Autodesk Inventor part; units mm, degrees
ref_plane "YZ Plane" through (0, 0, 0) normal (1, 0, 0) x (0, 1, 0)
ref_plane "XZ Plane" through (0, 0, 0) normal (0, 1, 0) x (-1, 0, 0)
ref_plane "XY Plane" through (0, 0, 0) normal (0, 0, 1) x (1, 0, 0)
sketch "Sketch1" plane through (0, 0, 0) normal (0, 1, 0) x (-1, 0, 0)
  line L0 (12.7, 25.4) -> (-12.7, 25.4)
  line L1 (-12.7, 25.4) -> (-12.7, -25.4)
  line L2 (-12.7, -25.4) -> (12.7, -25.4)
  line L3 (12.7, -25.4) -> (12.7, 25.4)
  line L4 (12.7, 25.4) -> (-12.7, -25.4) construction
  line L5 (-12.7, 25.4) -> (12.7, -25.4) construction
  point P0 (0, 0)
  dimension "d0" = 25.4
  dimension "d1" = 50.8
extrude "Extrusion1" add sketch "Sketch1" along normal blind 6.35
sketch "Sketch3" plane through (12.7, 0, 25.4) normal (1, 0, 0) x (0, 0, -1)
  line L0 (0, 6.35) -> (50.8, 6.35)
  line L1 (50.8, 6.35) -> (25.4, 6.35)
  line L2 (25.4, 6.35) -> (25.4, 0)
  line L3 (25.4, 0) -> (50.8, 0)
  line L4 (50.8, 0) -> (50.8, 6.35)
  dimension "d14" = 25.4
extrude "Extrusion2" add sketch "Sketch3" along normal blind 44.45
sketch "Sketch4" plane through (0, 6.35, 0) normal (0, 1, 0) x (1, 0, 0)
  line L0 (-12.7, -25.4) -> (12.7, -25.4)
  point P0 (0, 0)
  point P1 (0, -12.7)
  point P2 (0, 0)
  point P3 (0, 12.7)
  point P4 (0, -25.4)
  point P5 (0, -25.4)
  point P6 (0, -25.4)
  point P7 (25.4, 12.7)
  point P8 (38.1, 12.7)
  point P9 (50.8, 12.7)
  dimension "d17" = 12.7
  dimension "d18" = 12.7
  dimension "d19" = 12.7
  dimension "d20" = 25.4
  dimension "d21" = 12.7
  dimension "d22" = 12.7
hole "Hole2" at (0, 6.35, 12.7) at (0, 6.35, 0) at (0, 6.35, -12.7) at (25.4, 6.35, -12.7) at (38.1, 6.35, -12.7) at (50.8, 6.35, -12.7) direction (0, -1, 0) diameter 5.1054 end through all
fillet "Fillet1" radius 3.302 2 edges at (12.7, 3.175, 0) (-12.7, 3.175, -25.4)
properties part number "DB1-003" material "Aluminum 6061"
Source: CAD feature listing. Evaluate the final solid. Frame: model axes, mm. A direction names the side the tool comes from. Give positions to 0.01 mm unless a question says otherwise; leave off trailing zeros. Loops run counter-clockwise (first coordinate to the right, second up) from the corner with the lowest first, then second, coordinate; pieces in that order, holes last. Notation, with made-up numbers: (2.5, 9) -> (20.5, 9) arc R6 ccw to (20.5, 19) -> close; hole circle Ø9 at (-0.5, 83). An arc over 180 degrees is marked (long way). Use a Markdown table: item, result. Add a question column.
(1) First-contact query: pin 1 Ø3 at (y, z) = (4.5, 12) entering from +X; pin 2 Ø2 at (x, y) = (18, 4.5) entering from +Z. Flat tips, straight axial feed; report the tip coordinate or a pass-through.
(2) Pull-direction query (X, two-part tool) for faces 1 (the face through (12.7, 3, 15)), 2 (the face through (53.065, 3.131, -11.522)), 3 (the face through (15, 6.35, -5)), 4 (the face through (-12.7, 3, 1)); classes: +X half, -X half, draft (parallel to the pull), parting line (faces both ways), or undercut.
(3) Section query B-B (y = 2.5). Output: boundary loops of the cut face in (x, z), then the cut area to 3 significant figures.
(4) Ray query, line 1 (Z direction, x = 0, y = 3); line 2 (X direction, y = 3.25, z = -12.7); line 3 (X direction, y = 2.5, z = 12.7). Return the intervals inside material, ascending.
(5) Section query C-C (z = -12.7). Output: boundary loops of the cut face in (x, y), then the cut area to 3 significant figures.
(6) Section query A-A (x = 50.8). Output: boundary loops of the cut face in (y, z), then the cut area to 3 significant figures.
(7) Section query D-D (z = 12.7). Output: boundary loops of the cut face in (x, y), then the cut area to 3 significant figures.
(8) Access query for faces 5 (the face through (26.378, 3.131, -10.342)), 6 (the face through (36, 3, 0)). Directions: +Z, -Z, +X, -X, +Y, -Y. A direction counts if a zero-diameter tool reaches every point of the face in a straight line with its end or side. Return the directions, or none.
Checked values:
| question | item | result |
|---|---|---|
| 1 | pin 1 | x = 12.7 |
| 1 | pin 2 | z = 0 |
| 2 | face 1 | +X half |
| 2 | face 2 | undercut |
| 2 | face 3 | draft |
| 2 | face 4 | -X half |
| 3 | outline | (-12.7, -22.1) arc R3.3 ccw to (-9.4, -25.4) -> (57.15, -25.4) -> (57.15, 0) -> (16, 0) arc R3.3 cw to (12.7, 3.3) -> (12.7, 25.4) -> (-12.7, 25.4) -> close; hole circle Ø5.11 at (0, -12.7); hole circle Ø5.11 at (0, 0); hole circle Ø5.11 at (0, 12.7); hole circle Ø5.11 at (25.4, -12.7); hole circle Ø5.11 at (38.1, -12.7); hole circle Ø5.11 at (50.8, -12.7) |
| 3 | area | 2,300 mm^2 |
| 4 | line 1 | -25.4 to -15.25, -10.15 to -2.55, 2.55 to 10.15, 15.25 to 25.4 |
| 4 | line 2 | -12.7 to -2.55, 2.55 to 22.85, 27.95 to 35.55, 40.65 to 48.25, 53.35 to 57.15 |
| 4 | line 3 | -12.7 to -2.55, 2.55 to 12.7 |
| 5 | outline | (-12.7, 0) -> (-2.55, 0) -> (-2.55, 6.35) -> (-12.7, 6.35) -> close; (2.55, 0) -> (22.85, 0) -> (22.85, 6.35) -> (2.55, 6.35) -> close; (27.95, 0) -> (35.55, 0) -> (35.55, 6.35) -> (27.95, 6.35) -> close; (40.65, 0) -> (48.25, 0) -> (48.25, 6.35) -> (40.65, 6.35) -> close; (53.35, 0) -> (57.15, 0) -> (57.15, 6.35) -> (53.35, 6.35) -> close |
| 5 | area | 314 mm^2 |
| 6 | outline | (0, -25.4) -> (6.35, -25.4) -> (6.35, -15.25) -> (0, -15.25) -> close; (0, -10.15) -> (6.35, -10.15) -> (6.35, 0) -> (0, 0) -> close |
| 6 | area | 129 mm^2 |
| 7 | outline | (-12.7, 0) -> (-2.55, 0) -> (-2.55, 6.35) -> (-12.7, 6.35) -> close; (2.55, 0) -> (12.7, 0) -> (12.7, 6.35) -> (2.55, 6.35) -> close |
| 7 | area | 129 mm^2 |
| 8 | face 5 | +Y, -Y |
| 8 | face 6 | +Z, +X, +Y, -Y |
